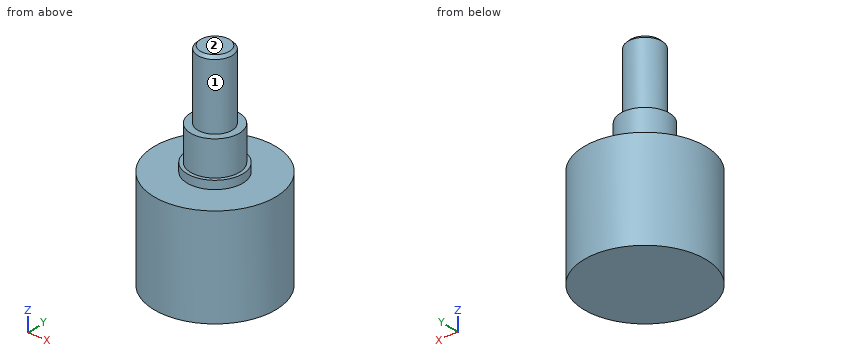
from build123d import *

# Parameters (mm, degrees)
SKETCH1_R       = 11.2395
BODY_DEPTH      = 18.446
SKETCH2_R       = 5.1435
LIP_DEPTH       = 1.524
SKETCH3_R       = 4.5
THREADING_DEPTH = 6.396
SKETCH4_R       = 3.175
SHAFT_DEPTH     = 20.617
CHAMFER1_SIZE   = 0.508


with BuildPart() as part:
    # Sketch1 → Body (new body)
    with BuildSketch(Plane.XY):
        Circle(SKETCH1_R)
    extrude(amount=BODY_DEPTH)

    # Sketch2 → Lip (add)
    with BuildSketch(Plane.XY.offset(18.446)):
        with Locations(Location((0, 0, 0), (0, 0, 180))):
            Circle(SKETCH2_R)
    extrude(amount=LIP_DEPTH)

    # Sketch3 → Threading (add)
    with BuildSketch(Plane.XY.offset(19.97)):
        Circle(SKETCH3_R)
    extrude(amount=THREADING_DEPTH)

    # Sketch4 → Shaft (add)
    with BuildSketch(Plane.XY.offset(18.446)):
        Circle(SKETCH4_R)
    extrude(amount=SHAFT_DEPTH)

    # Chamfer1
    chamfer1_edges = [part.edges().sort_by_distance(p)[0] for p in [
        (-3.175, 0, 39.063),
    ]]
    chamfer(chamfer1_edges, length=CHAMFER1_SIZE)


solid = part.part
Design review of the part built by this model. Coordinates are the model's own, in mm. Face numbers are marked on the shaded views. A direction names the side the tool comes from. Coordinates: 2 decimals unless noted, no trailing zeros. Order: outer loops, then holes, each group sorted by start corner. A loop starts at its lowest first (then second) coordinate and runs counter-clockwise, first axis right, second up. Notation, with made-up numbers: (69.25, 59.25) -> (96.25, 59.25) arc R34 cw to (96.25, 95.25) -> close; hole circle Ø2 at (-5, -7.75). An arc over 180 degrees is marked (long way). Use one line per item in the form item = value. Start each with the question number.
(1) Insertion check: pin 1 (12 mm diameter, centred on x = -1.5, z = 32, fed in from +Y); pin 2 (1.5 mm diameter, centred on x = -6, y = 2.5, fed in from +Z); pin 3 (6 mm diameter, centred on x = -6, z = 8, fed in from -Y); pin 4 (3 mm diameter, centred on y = 5.5, z = 29, fed in from -X). Each pin has a flat end and moves straight along its axis. Give the tip position at first contact, or say it passes through.
(2) Add section D-D on z = 30. State the section outline as (x, y) points (3 decimals), plus the area to 3 significant figures.
(3) For the marked faces 1 and 2, list the 3-axis set-ups (+Z, -Z, +X, -X, +Y, -Y) from which the entire face can be reached by the end or side of a thin tool; tool diameter is ignored.
(4) Add section C-C on z = 12.5. State the section outline as (x, y) points, plus the area to 3 significant figures.
(5) Add section A-A on y = 0. State the section outline as (x, z) points (1 decimal), plus the area to 3 significant figures.
(6) For probe 1 along Z at (x, y) = (6.5, 8); probe 2 along Y at (x, z) = (-0.25, 32.5); probe 3 along Z at (x, y) = (-2.5, -2.25), list the stretches that pass through material, from the lowest coordinate up.
Answer block:
q1.pin_1 = 4.5
q1.pin_2 = 18.45
q1.pin_3 = -10.83
q1.pin_4 = through
q2.outline = circle Ø6.35 at (0, 0)
q2.area = 31.7 mm²
q3.face_1 = +Z
q3.face_2 = +Z, +X, -X, +Y, -Y
q4.outline = circle Ø22.48 at (0, 0)
q4.area = 397 mm²
q5.outline = (-11.2, 0) -> (11.2, 0) -> (11.2, 18.4) -> (5.1, 18.4) -> (5.1, 20) -> (4.5, 20) -> (4.5, 26.4) -> (3.2, 26.4) -> (3.2, 38.6) -> (2.7, 39.1) -> (-2.7, 39.1) -> (-3.2, 38.6) -> (-3.2, 26.4) -> (-4.5, 26.4) -> (-4.5, 20) -> (-5.1, 20) -> (-5.1, 18.4) -> (-11.2, 18.4) -> close
q5.area = 568 mm²
q6.probe_1 = 0 to 18.45
q6.probe_2 = -3.17 to 3.17
q6.probe_3 = 0 to 26.37
